```python
from build123d import *

# Parameters (mm, degrees)
SKETCH1_W           = 91.44
SKETCH1_H           = 60.452
BOSS_EXTRUDE1_DEPTH = 8.89
SKETCH2_W           = 81.28
SKETCH2_H           = 57.15
CUT_EXTRUDE1_DEPTH  = 1.6002
SKETCH3_R           = 6.35
SKETCH3_R_2         = 1.28905
CUT_EXTRUDE2_DEPTH  = 4.7498
SKETCH4_R           = 1.28905
CUT_EXTRUDE3_DEPTH  = 56.524423239
CUT_EXTRUDE4_REACH  = 78.314
SKETCH5_W           = 3.9116
SKETCH5_H           = 0.8636


with BuildPart() as part:
    # Sketch1 → Boss-Extrude1 (new body)
    with BuildSketch(Plane(origin=(0, 0, 0), x_dir=(1, 0, 0), z_dir=(0, 1, 0))):
        Rectangle(SKETCH1_W, SKETCH1_H)
    extrude(amount=BOSS_EXTRUDE1_DEPTH)

    # Sketch2 → Cut-Extrude1 (cut)
    with BuildSketch(Plane(origin=(0, 8.89, 0), x_dir=(1, 0, 0), z_dir=(0, 1, 0))):
        Rectangle(SKETCH2_W, SKETCH2_H)
    extrude(amount=-CUT_EXTRUDE1_DEPTH, mode=Mode.SUBTRACT)

    # Sketch3 → Cut-Extrude2 (cut)
    with BuildSketch(Plane(origin=(0, 7.2898, 0), x_dir=(1, 0, 0), z_dir=(0, 1, 0))):
        Polygon((-40.64, 28.575), (27.94, 28.575), (27.94, 15.875), (40.64, 15.875), (40.64, -22.225), (-27.94, -22.225), (-27.94, -28.575), (-40.64, -28.575), (-40.64, -22.225), align=None)
        with Locations(Location((-14.351, 8.255, 0), (0, 0, 270))):
            Circle(SKETCH3_R, mode=Mode.SUBTRACT)
        with Locations(Location((-14.351, 8.255, 0), (0, 0, 270))):
            Circle(SKETCH3_R_2)
    extrude(amount=-CUT_EXTRUDE2_DEPTH, mode=Mode.SUBTRACT)

    # Sketch4 → Cut-Extrude3 (cut, through all)
    with BuildSketch(Plane(origin=(0, 8.89, 0), x_dir=(1, 0, 0), z_dir=(0, 1, 0))):
        with Locations(Location((-42.545, 27.051, 0), (0, 0, 270))):
            Circle(SKETCH4_R)
        with Locations(Location((-42.545, -27.051, 0), (0, 0, 270))):
            Circle(SKETCH4_R)
        with Locations(Location((42.545, -27.051, 0), (0, 0, 270))):
            Circle(SKETCH4_R)
        with Locations(Location((42.545, 27.051, 0), (0, 0, 270))):
            Circle(SKETCH4_R)
    extrude(amount=-CUT_EXTRUDE3_DEPTH, mode=Mode.SUBTRACT)

    # Sketch5 → Cut-Extrude4 (cut, up to next)
    with BuildSketch(Plane(origin=(0, 0, -30.226), x_dir=(-1, 0, 0), z_dir=(0, 0, -1)), mode=Mode.PRIVATE) as cut_extrude4_sk1:
        with Locations((-4.699, 8.4582)):
            Rectangle(SKETCH5_W, SKETCH5_H)
    cut_extrude4_tool1 = extrude(cut_extrude4_sk1.sketch, amount=-CUT_EXTRUDE4_REACH, mode=Mode.PRIVATE) & part.part
    add(cut_extrude4_tool1.solids().sort_by_distance((4.699, 8.4582, -30.226))[0], mode=Mode.SUBTRACT)


solid = part.part
```
Check sheet for the modelled part. Datum: model origin and axes. Units: mm. A direction names the side the tool comes from. Round coordinates to 2 decimals unless told otherwise and drop trailing zeros. Order: outer loops, then holes, each group sorted by start corner. A loop starts at its lowest first (then second) coordinate and runs counter-clockwise, first axis right, second up. Notation, with made-up numbers: (59, 30) -> (110, 30) arc R35 cw to (110, 69) -> close; hole circle Ø9 at (87, 35.25). An arc over 180 degrees is marked (long way). Use CSV: the item, a comma, the result in double quotes.
(1) Tool access check on faces 4 (the face through (-45.72, 4, 0)), 5 (the face through (-27.94, 5, 25)). Record the directions out of +Z, -Z, +X, -X, +Y, -Y that give a thin tool (end or side, any length) a straight path to the whole face; none if there is none.
Worked out:
face 4,"+Z, -Z, -X, +Y, -Y"
face 5,"+Y"
(2) Depth check by flat-ended pin: pin 1 (12 mm diameter, centred on x = -7, z = 13, fed in from +Y); pin 2 (2.5 mm diameter, centred on x = -42.545, z = -27.051, fed in from -Y); pin 3 (3 mm diameter, centred on x = -14, z = -8, fed in from +Y); pin 4 (0.5 mm diameter, centred on x = 5.5, z = -29, fed in from +Y). Enter the tip coordinate at first touch or a pass-through.
Worked out:
pin 1,"y = 2.54"
pin 2,"through"
pin 3,"y = 7.29"
pin 4,"y = 8.03"
(3) Cross-section at A-A (y = 5). Record the boundary of the cut face in (x, z) (3 decimals), and give its area (3 significant figures).
Worked out:
outline,"(-45.72, -30.226) -> (45.72, -30.226) -> (45.72, 30.226) -> (-45.72, 30.226) -> close; circle Ø12.7 at (-14.351, -8.255); hole circle Ø2.578 at (-42.545, -27.051); hole circle Ø2.578 at (-42.545, 27.051); hole (-40.64, -28.575) -> (27.94, -28.575) -> (27.94, -15.875) -> (40.64, -15.875) -> (40.64, 22.225) -> (-27.94, 22.225) -> (-27.94, 28.575) -> (-40.64, 28.575) -> close; hole circle Ø2.578 at (-14.351, -8.255); hole circle Ø2.578 at (42.545, -27.051); hole circle Ø2.578 at (42.545, 27.051)"
area,"1,580 mm²"
(4) Cross-section at B-B (x = 36.5). Record the boundary of the cut face in (y, z) (3 decimals), and give its area (3 significant figures).
Worked out:
outline,"(0, -30.226) -> (8.89, -30.226) -> (8.89, -28.575) -> (7.29, -28.575) -> (7.29, -15.875) -> (2.54, -15.875) -> (2.54, 22.225) -> (7.29, 22.225) -> (7.29, 28.575) -> (8.89, 28.575) -> (8.89, 30.226) -> (0, 30.226) -> close"
area,"265 mm²"
(5) Draft check along Z on faces 1 (the face through (-43.803, 4.507, -27.33)), 2 (the face through (-1, 4, -30.226)), 3 (the face through (45.72, 4, 0)). Enter one of: pulls with the +Z half, pulls with the -Z half, needs draft (parallel to the pull), parting line crosses it, or undercut.
Worked out:
face 1,"undercut"
face 2,"pulls with the -Z half"
face 3,"needs draft"
(6) Cross-section at D-D (z = 1.5). Record the boundary of the cut face in (x, y).
Worked out:
outline,"(-45.72, 0) -> (45.72, 0) -> (45.72, 8.89) -> (40.64, 8.89) -> (40.64, 2.54) -> (-40.64, 2.54) -> (-40.64, 8.89) -> (-45.72, 8.89) -> close"
(7) Material ranges on line 1 along Z through (x, y) = (18.5, 4) (3 decimals); line 2 along X through (y, z) = (7, 21.5); line 3 along X through (y, z) = (4, -25), recorded low to high. Write a range as from..to.
Worked out:
line 1,"-30.226..-28.575, 22.225..30.226"
line 2,"-45.72..-40.64, 40.64..45.72"
line 3,"-45.72..-40.64, 27.94..45.72"
(8) Cross-section at C-C (z = -23). Record the boundary of the cut face in (x, y), and give its area (3 significant figures).
Worked out:
outline,"(-45.72, 0) -> (45.72, 0) -> (45.72, 8.89) -> (40.64, 8.89) -> (40.64, 7.29) -> (27.94, 7.29) -> (27.94, 2.54) -> (-40.64, 2.54) -> (-40.64, 8.89) -> (-45.72, 8.89) -> close"
area,"357 mm²"
